from build123d import *

# Parameters (mm, degrees)
SKETCH_R     = 4
PAD_DEPTH    = 30
SKETCH001_R  = 2
POCKET_DEPTH = 5


with BuildPart() as part:
    # Sketch → Pad (new body)
    with BuildSketch(Plane.XZ):
        Polygon((-17, -11), (-17, -5), (-15, -3), (-15, 7), (-8, 7), (-4, 11), (4, 11), (8, 7), (15, 7), (15, -3), (17, -5), (17, -11), align=None)
        Circle(SKETCH_R, mode=Mode.SUBTRACT)
    extrude(amount=PAD_DEPTH)

    # Sketch001 (on Face12 of Pad) → Pocket (cut)
    with BuildSketch(Plane(origin=(0, 0, -11), x_dir=(1, 0, 0), z_dir=(0, 0, -1))):
        with Locations((-12, 24)):
            Circle(SKETCH001_R)
        with Locations((12, 24)):
            Circle(SKETCH001_R)
        with Locations((-12, 6)):
            Circle(SKETCH001_R)
        with Locations((12, 6)):
            Circle(SKETCH001_R)
    extrude(amount=-POCKET_DEPTH, mode=Mode.SUBTRACT)


solid = part.part
Model file for the job. Use its own axes, mm. A direction names the side the tool comes from. Give positions to 0.01 mm unless a question says otherwise; leave off trailing zeros. Loops run counter-clockwise (first coordinate to the right, second up) from the corner with the lowest first, then second, coordinate; pieces in that order, holes last. Notation, with made-up numbers: (-4.5, 69) - (14.5, 69) arc R37 cw to (14.5, 106) - close; hole circle Ø8 at (18, -23.5). An arc over 180 degrees is marked (long way). Use one line per item in the form item = value.
(1) Cut at A-A (z = 0). Give the cut face in (x, y).
Determined:
outline = (-15, -30) - (-4, -30) - (-4, 0) - (-15, 0) - close; (4, -30) - (15, -30) - (15, 0) - (4, 0) - close
(2) 3-axis set-ups, long thin cutter, end or side, ignore diameter. For faces 1 (the face through (0, -15, 11)), 2 (the face through (-15, -15, 2)), 3 (the face through (10, -6, -9)), 4 (the face through (11, -15, 7)): which of +Z, -Z, +X, -X, +Y, -Y reach the whole face in a straight line?
Determined:
face_1 = +Z, +X, -X, +Y, -Y
face_2 = +Z, -X, +Y, -Y
face_3 = -Z
face_4 = +Z, +X, +Y, -Y
(3) Drop flat-ended pins along their axis: P1, Ø7.5, axis at x = 10.5, y = -15, coming from the +Z side; P2, Ø6, axis at y = -10, z = -4.5, coming from the -X side; P3, Ø7, axis at x = 0, z = 0, coming from the -Y side (3 decimals); P4, Ø8, axis at y = -21, z = -0.5, coming from the -X side. Give the stop position or say it passes through.
Determined:
P1 = 8.25
P2 = -17
P3 = through
P4 = -16.5
(4) Drill centre lines: L1, parallel to Y at x = 12, z = -8.4; L2, parallel to X at y = -24, z = -9.4; L3, parallel to Z at x = 0, y = -22.75. Where is each one in solid material? Low to high.
Determined:
L1 = -30 to -26, -22 to -8, -4 to 0
L2 = -17 to -14, -10 to 10, 14 to 17
L3 = -11 to -4, 4 to 11
(5) Cut at C-C (x = 0). Give the cut face in (y, z).
Determined:
outline = (-30, -11) - (0, -11) - (0, -4) - (-30, -4) - close; (-30, 4) - (0, 4) - (0, 11) - (-30, 11) - close
(6) Cut at D-D (x = 12). Give the cut face in (y, z).
Determined:
outline = (-30, -11) - (-26, -11) - (-26, -6) - (-22, -6) - (-22, -11) - (-8, -11) - (-8, -6) - (-4, -6) - (-4, -11) - (0, -11) - (0, 7) - (-30, 7) - close
(7) Pull direction Y, two halves, no side cores. Call faces 5 (the face through (-4, -30, -2)), 6 (the face through (-17, -15, -8)), 7 (the face through (-13.474, -7.352, -8.535)): pulls with the +Y half, pulls with the -Y half, needs draft (parallel to the pull), parting line crosses it, or undercut.
Determined:
face_5 = pulls with the -Y half
face_6 = needs draft
face_7 = undercut
(8) Cut at B-B (y = -6). Give the cut face in (x, z).
Determined:
outline = (-17, -11) - (-14, -11) - (-14, -6) - (-10, -6) - (-10, -11) - (10, -11) - (10, -6) - (14, -6) - (14, -11) - (17, -11) - (17, -5) - (15, -3) - (15, 7) - (8, 7) - (4, 11) - (-4, 11) - (-8, 7) - (-15, 7) - (-15, -3) - (-17, -5) - close; hole circle Ø8 at (0, 0)
